from build123d import *

# Parameters (mm, degrees)
SKETCH1_W           = 32.004
SKETCH1_H           = 32.004
BOSS_EXTRUDE1_DEPTH = 1.5748
SKETCH2_W           = 20.32
SKETCH2_H           = 20.32
BOSS_EXTRUDE2_DEPTH = 5.7404
SKETCH3_R           = 7.3914
BOSS_EXTRUDE3_DEPTH = 15.9512
SKETCH4_R           = 1.0668
CUT_EXTRUDE1_DEPTH  = 15.9512
SKETCH5_R           = 3.81
CUT_EXTRUDE2_DEPTH  = 2.032
CHAMFER1_SIZE       = 2.794
DOME2_FACE_RADIUS   = 4.572
DOME2_HEIGHT        = 2.54


with BuildPart() as part:
    # Sketch1 → Boss-Extrude1 (new body)
    with BuildSketch(Plane.XY):
        Rectangle(SKETCH1_W, SKETCH1_H)
    extrude(amount=BOSS_EXTRUDE1_DEPTH)

    # Sketch2 → Boss-Extrude2 (add)
    with BuildSketch(Plane.XY.offset(1.5748)):
        Rectangle(SKETCH2_W, SKETCH2_H)
    extrude(amount=BOSS_EXTRUDE2_DEPTH)

    # Sketch3 → Boss-Extrude3 (add)
    with BuildSketch(Plane.XY.offset(7.3152)):
        Circle(SKETCH3_R)
    extrude(amount=BOSS_EXTRUDE3_DEPTH)

    # Sketch4 → Cut-Extrude1 (cut)
    with BuildSketch(Plane.XY.offset(1.5748)):
        with Locations((-13.9192, 13.9192)):
            Circle(SKETCH4_R)
        with Locations((-13.9192, -13.9192)):
            Circle(SKETCH4_R)
        with Locations((13.9192, 13.9192)):
            Circle(SKETCH4_R)
        with Locations((13.9192, -13.9192)):
            Circle(SKETCH4_R)
    extrude(amount=-CUT_EXTRUDE1_DEPTH, mode=Mode.SUBTRACT)

    # Sketch5 → Cut-Extrude2 (cut)
    with BuildSketch(Plane.XY.offset(23.2664)):
        Circle(SKETCH5_R)
    extrude(amount=-CUT_EXTRUDE2_DEPTH, mode=Mode.SUBTRACT)

    # Chamfer1
    # the kernel refuses this chamfer: 2.794 mm, written as the material it takes off along each edge
    with BuildSketch(Plane(origin=(0, 0, 23.2664), x_dir=(1, 0, 0), z_dir=(0, -1, 0))) as chamfer1_piece_1_section:
        Polygon((3.81 + CHAMFER1_SIZE, 0), (3.81, -CHAMFER1_SIZE), (3.81, 0), align=None)
    chamfer1_piece_1 = revolve(axis=Axis((0, 0, 23.2664), (0, 0, 1)), mode=Mode.PRIVATE)
    chamfer1_piece_1 = split(chamfer1_piece_1, bisect_by=Plane(origin=(-5.592803541, 0, 21.2344), z_dir=(0, 0, 1)), keep=Keep.TOP, mode=Mode.PRIVATE)
    add(chamfer1_piece_1, mode=Mode.SUBTRACT)

    # Dome2: a dome of height H over a round flat face of radius A is a cap of a sphere of radius (A * A + H * H) / (2 * H)
    dome2_r = (DOME2_FACE_RADIUS * DOME2_FACE_RADIUS + DOME2_HEIGHT * DOME2_HEIGHT) / (2 * DOME2_HEIGHT)
    dome2_base = Plane((0, 0, 21.2344), z_dir=(0, 0, 1))
    with Locations(dome2_base.offset(DOME2_HEIGHT - dome2_r)):
        dome2_ball = Sphere(dome2_r, mode=Mode.PRIVATE)
    add(split(dome2_ball, bisect_by=dome2_base, keep=Keep.TOP, mode=Mode.PRIVATE))


solid = part.part
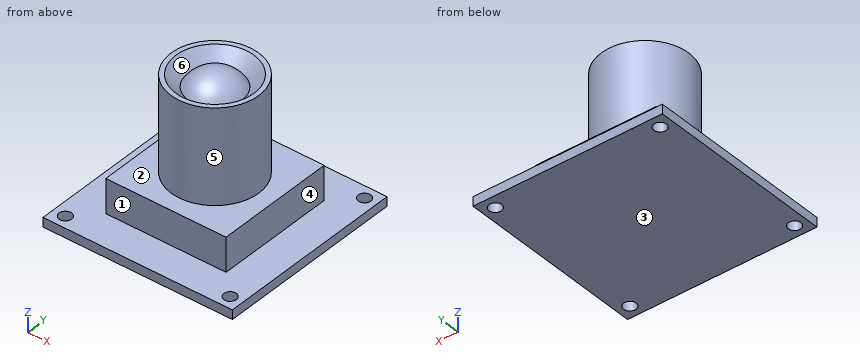
Geometry check sheet. Reference: the model listing, model coordinates, mm. Face numbers are marked on the shaded views. A direction names the side the tool comes from. Round coordinates to 2 decimals unless told otherwise and drop trailing zeros. Order: outer loops, then holes, each group sorted by start corner. A loop starts at its lowest first (then second) coordinate and runs counter-clockwise, first axis right, second up. Notation, with made-up numbers: M -30,88 L 29,88 A38 cw 29,127 Z; hole C 36,78.5 d1. An arc over 180 degrees is marked long. Answer in a Markdown table with one row per item.
(1) Scan lines: probe 1 along Z at (x, y) = (-7, -11.5); probe 2 along Y at (x, z) = (0, 2). Record each from-to range of solid material in increasing order. Write a range as from..to.
Responses:
| item | result |
|---|---|
| probe 1 | z = 0..1.57 |
| probe 2 | y = -10.16..10.16 |
(2) Sectioned sample at D-D, the plane z = 4.5. Record the cut outline in (x, y), and give its area (3 significant figures).
Responses:
| item | result |
|---|---|
| outline | M -10.16,-10.16 L 10.16,-10.16 L 10.16,10.16 L -10.16,10.16 Z |
| area | 413 mm² |
(3) Tool access check on the marked faces 1, 2 and 3. Record the directions out of +Z, -Z, +X, -X, +Y, -Y that give a thin tool (end or side, any length) a straight path to the whole face; none if there is none.
Responses:
| item | result |
|---|---|
| face 1 | +Z, +X, -X, -Y |
| face 2 | +Z |
| face 3 | -Z, +X, -X, +Y, -Y |
(4) Draft check along Y on the marked faces 4, 5 and 6. Enter one of: released by +Y, released by -Y, zero draft, split by the parting line, or undercut.
Responses:
| item | result |
|---|---|
| face 4 | zero draft |
| face 5 | split by the parting line |
| face 6 | undercut |
(5) Sectioned sample at A-A, the plane y = 0. Record the cut outline in (x, z), and give its area (3 significant figures).
Responses:
| item | result |
|---|---|
| outline | M -16,0 L 16,0 L 16,1.57 L 10.16,1.57 L 10.16,7.32 L 7.39,7.32 L 7.39,23.27 L 6.6,23.27 L 4.57,21.23 A5.38 ccw -4.57,21.23 L -6.6,23.27 L -7.39,23.27 L -7.39,7.32 L -10.16,7.32 L -10.16,1.57 L -16,1.57 Z |
| area | 397 mm² |
(6) Go/stop test with flat-tipped pins: P1, Ø1, axis at y = -5.5, z = 19, coming from the -X side; P2, Ø4, axis at x = 9.5, y = 4, coming from the -Z side; P3, Ø12, axis at x = 6, y = 9, coming from the +Z side; P4, Ø1.3, axis at x = 13.92, y = -13.92, coming from the +Z side. Record where each tip stops, or that it passes through.
Responses:
| item | result |
|---|---|
| P1 | stops at x = -5.44 |
| P2 | stops at z = 0 |
| P3 | stops at z = 23.27 |
| P4 | passes through |
(7) Sectioned sample at B-B, the plane x = 13.5. Record the cut outline in (y, z), and give its area (3 significant figures).
Responses:
| item | result |
|---|---|
| outline | M -16,0 L -14.9,0 L -14.9,1.57 L -16,1.57 Z; M -12.94,0 L 12.94,0 L 12.94,1.57 L -12.94,1.57 Z; M 14.9,0 L 16,0 L 16,1.57 L 14.9,1.57 Z |
| area | 44.2 mm² |
